from build123d import *

# Parameters (mm, degrees)
F0_W          = 3
F0_H          = 3
F0_W_2        = 4.5
F0_W_3        = 25
F1_DEPTH      = 10
F1_DEPTH_BACK = 10
F4_DEPTH      = 10
F4_DEPTH_BACK = 10
F5_R          = 6


with BuildPart() as f1:
    # F0 (on Front) → F1 (new body, two sides)
    with BuildSketch(Plane.XZ) as f1_sk:
        with Locations((1.5, 1.5)):
            Rectangle(F0_W, F0_H)
        Polygon((3, 0), (0, 0), (0, -22), (0, -25), (3, -25), align=None)
        with Locations((5.25, 1.5)):
            Rectangle(F0_W_2, F0_H)
        with Locations((-12.5, -23.5)):
            Rectangle(F0_W_3, F0_H)
        Polygon((7.5, 3), (7.5, 0), (7.5, -25), (10.5, -25), (10.5, 3), align=None)
    extrude(amount=F1_DEPTH)
    extrude(f1_sk.sketch, amount=-F1_DEPTH_BACK)

    # F3 (on offset) → F4 (cut, two sides)
    with BuildSketch(Plane.XY.offset(-20)) as f4_sk:
        with BuildLine():
            ThreePointArc((-15, -5), (-11.464466, -3.535534), (-10, 0))
            Line((-10, 0), (-25, 0))
            Line((-25, 0), (-25, -5))
            Line((-25, -5), (-15, -5))
        make_face()
        with BuildLine():
            Line((-25, 0), (-10, 0))
            ThreePointArc((-10, 0), (-11.464466, 3.535534), (-15, 5))
            Line((-15, 5), (-25, 5))
            Line((-25, 5), (-25, 0))
        make_face()
    extrude(amount=F4_DEPTH, mode=Mode.SUBTRACT)
    extrude(f4_sk.sketch, amount=-F4_DEPTH_BACK, mode=Mode.SUBTRACT)

    # F5
    f5_edges = [f1.edges().sort_by_distance(p)[0] for p in [
        (0, 0, -22),
    ]]
    fillet(f5_edges, radius=F5_R)


solid = f1.part
Could you check a few things on this model? Use its own coordinates, in mm. A direction names the side the tool comes from. Give positions to 0.01 mm unless a question says otherwise; leave off trailing zeros. Order: outer loops, then holes, each group sorted by start corner. A loop starts at its lowest first (then second) coordinate and runs counter-clockwise, first axis right, second up. Notation, with made-up numbers: (-22.5, 26.5) -> (3.5, 26.5) arc R11 cw to (3.5, 43.5) -> close; hole circle Ø4 at (-15.75, -32.75). An arc over 180 degrees is marked (long way). Return JSON: item names as keys, results as strings.
1. On a 3-axis mill with a long thin cutter (end or side, diameter ignored), from which of +Z, -Z, +X, -X, +Y, -Y can I reach the whole of each face in a straight line? I mean faces 1 (the flat face through (0, 0, -6)), 2 (the flat face through (1, 10, -15)), 3 (the flat face through (7.5, 0, -12)), 4 (the flat face through (-20, -5, -23)), 5 (the flat face through (-8, 0, -25)). Say none if no direction works.
Answer list:
{"face 1": "+Z, -X, +Y, -Y", "face 2": "+Z, -Z, +X, -X, +Y", "face 3": "-Z, +Y, -Y", "face 4": "+Z, -Z, -X", "face 5": "-Z, +X, -X, +Y, -Y"}
2. Imagine slicing it at D-D on z = -11.25. List the corners of the cut face in (x, y) for me, then the cut area to 3 significant figures.
Answer list:
{"outline": "(0, -10) -> (3, -10) -> (3, 10) -> (0, 10) -> close; (7.5, -10) -> (10.5, -10) -> (10.5, 10) -> (7.5, 10) -> close", "area": "120 mm2"}
3. Imagine slicing it at A-A on z = -22.75. List the corners of the cut face in (x, y) for me, then the cut area to 3 significant figures.
Answer list:
{"outline": "(-25, -10) -> (3, -10) -> (3, 10) -> (-25, 10) -> (-25, 5) -> (-15, 5) arc R5 cw to (-15, -5) -> (-25, -5) -> close; (7.5, -10) -> (10.5, -10) -> (10.5, 10) -> (7.5, 10) -> close", "area": "481 mm2"}
4. I need wall thicknesses on line 1 (X direction, y = -2.25, z = -16); line 2 (Z direction, x = -20, y = -6.75); line 3 (X direction, y = 2.75, z = 1.25). Which ranges of each line are inside material? Lowest first, please. Write a range as from..to.
Answer list:
{"line 1": "x = 0..3, 7.5..10.5", "line 2": "z = -25..-22", "line 3": "x = 0..10.5"}
5. Thinking about a two-plate mould opening in Y: for faces 6 (the flat face through (1, -10, -15)), 7 (the flat face through (5, 0, 3)), 8 (the flat face through (-20, 5, -23)), which applies, pulls with the +Y half, pulls with the -Y half, needs draft (parallel to the pull), parting line crosses it, or undercut?
Answer list:
{"face 6": "pulls with the -Y half", "face 7": "needs draft", "face 8": "undercut"}
6. Imagine slicing it at B-B on x = -19. List the corners of the cut face in (y, z) for me.
Answer list:
{"outline": "(-10, -25) -> (-5, -25) -> (-5, -22) -> (-10, -22) -> close; (5, -25) -> (10, -25) -> (10, -22) -> (5, -22) -> close"}
7. Imagine slicing it at C-C on y = 5.75. List the corners of the cut face in (x, z) for me.
Answer list:
{"outline": "(-25, -25) -> (3, -25) -> (3, 0) -> (7.5, 0) -> (7.5, -25) -> (10.5, -25) -> (10.5, 3) -> (0, 3) -> (0, -16) arc R6 cw to (-6, -22) -> (-25, -22) -> close"}
8. For pin 1 Ø1.5 at (x, z) = (4, -4) entering from +Y; pin 2 Ø1 at (y, z) = (1, -1) entering from -X; pin 3 Ø10 at (x, y) = (-9, 0) entering from +Z, each with a flat end and sliding along its axis, tell me the tip position at first contact or that it passes through.
Answer list:
{"pin 1": "passes through", "pin 2": "stops at x = 0", "pin 3": "stops at z = -21.66"}
